Can you work these out from the model? Positions are in its coordinate system, mm. Face numbers are marked on the shaded views. A direction names the side the tool comes from. Give positions to 0.01 mm unless a question says otherwise; leave off trailing zeros. Order: outer loops, then holes, each group sorted by start corner. A loop starts at its lowest first (then second) coordinate and runs counter-clockwise, first axis right, second up. Notation, with made-up numbers: (-7.5, 55) - (43.5, 55) arc R34 ccw to (43.5, 87) - close; hole circle Ø9 at (44.25, 56). An arc over 180 degrees is marked (long way). Return JSON: item names as keys, results as strings.
Autodesk Inventor part; units mm, degrees
ref_plane "YZ Plane" through (0, 0, 0) normal (1, 0, 0) x (0, 1, 0)
ref_plane "XZ Plane" through (0, 0, 0) normal (0, 1, 0) x (-1, 0, 0)
ref_plane "XY Plane" through (0, 0, 0) normal (0, 0, 1) x (1, 0, 0)
sketch "Sketch1" plane through (0, 0, 0) normal (0, 0, 1) x (1, 0, 0)
  circle A0 centre (50.3282, 23.2015) radius 3
  circle A1 centre (18.8282, 23.2015) radius 3
  circle A2 centre (34.5782, 23.2015) radius 4
  arc A3 (37.4648, 32.7758) -> (30.5806, 32.3677) centre (34.5782, 23.2015) ccw
  arc A4 (50.3282, 17.7015) -> (51.8996, 28.4722) centre (50.3282, 23.2015) ccw
  line L0 (37.4648, 32.7758) -> (51.8996, 28.4722)
  line L1 (34.3282, 9.7015) -> (44.1532, 9.7015)
  line L2 (44.1532, 9.7015) -> (44.1532, 16.7015)
  line L3 (44.1532, 16.7015) -> (50.3282, 17.7015)
  line L4 (30.5806, 32.3677) -> (17.2831, 28.48)
  line L5 (34.3282, 9.7015) -> (25.0032, 9.7015)
  line L6 (25.0032, 9.7015) -> (25.0032, 16.7015)
  line L7 (25.0032, 16.7015) -> (18.8282, 17.7015)
  arc A5 (17.2831, 28.48) -> (18.8282, 17.7015) centre (18.8282, 23.2015) ccw
  circle A6 centre (34.5782, 23.2015) radius 8.7313
  point P0 (0, 0)
  dimension "d0" = 31.5
  dimension "d1" = 6
  dimension "d2" = 8
  dimension "d3" = 15.75
  dimension "d4" = 20
  dimension "d5" = 11
  dimension "d7" = 9.825
  dimension "d8" = 7
  dimension "d9" = 11
  dimension "d12" = 17.4625
  dimension "d14" = 0
extrude "Extrusion1" add sketch "Sketch1" along normal blind 10 contours L0 A4 L3 L2 L1 L5 L6 L7 A5 L4 A3 | A6
properties part number "shaft support"
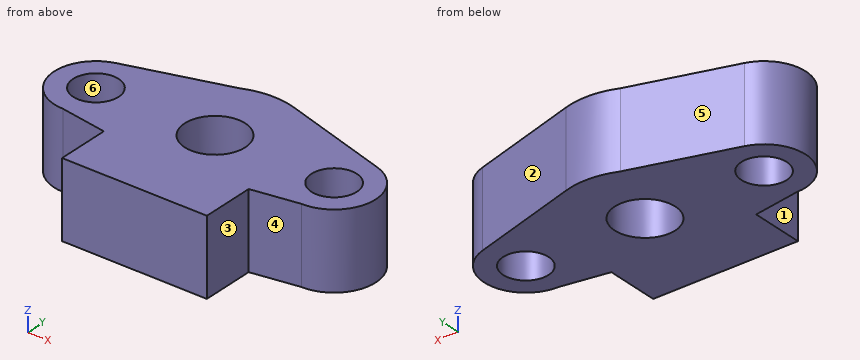
1. Thinking about a two-plate mould opening in X: for the marked faces 4, 5 and 6, which applies, +X half, -X half, draft (parallel to the pull), parting line (faces both ways), or undercut?
Checks:
{"face 4": "+X half", "face 5": "-X half", "face 6": "undercut"}
2. Suppose I cut it at D-D (y = 14.25). List the corners of the cut face in (x, z) for me.
Checks:
{"outline": "(25, 0) - (44.15, 0) - (44.15, 10) - (25, 10) - close"}
3. Suppose I cut it at C-C (y = 21.75). List the corners of the cut face in (x, z) for me, plus the area to 3 significant figures.
Checks:
{"outline": "(13.52, 0) - (16.2, 0) - (16.2, 10) - (13.52, 10) - close; (21.45, 0) - (30.85, 0) - (30.85, 10) - (21.45, 10) - close; (38.31, 0) - (47.7, 0) - (47.7, 10) - (38.31, 10) - close; (52.95, 0) - (55.63, 0) - (55.63, 10) - (52.95, 10) - close", "area": "242 mm^2"}
4. Suppose I cut it at B-B (z = 6). List the corners of the cut face in (x, y) for me, plus the area to 3 significant figures.
Checks:
{"outline": "(17.28, 28.48) arc R5.5 ccw to (18.83, 17.7) - (25, 16.7) - (25, 9.7) - (44.15, 9.7) - (44.15, 16.7) - (50.33, 17.7) arc R5.5 ccw to (51.9, 28.47) - (37.46, 32.78) arc R10 ccw to (30.58, 32.37) - close; hole circle Ø6 at (18.83, 23.2); hole circle Ø8 at (34.58, 23.2); hole circle Ø6 at (50.33, 23.2)", "area": "574 mm^2"}
5. For pin 1 Ø5 at (y, z) = (29.5, 4) entering from +X; pin 2 Ø5.5 at (y, z) = (13, 7) entering from +X; pin 3 Ø5.5 at (y, z) = (12, 4.5) entering from -X, each with a flat end and sliding along its axis, tell me the tip position at first contact or that it passes through.
Checks:
{"pin 1": "x = 54.31", "pin 2": "x = 44.15", "pin 3": "x = 25"}
6. If I drill on L1, parallel to X at y = 23.25, z = 1; L2, parallel to X at y = 25, z = 4.5; L3, parallel to Y at x = 35, z = 8, over which ranges is the centre line in solid material (lowest first)? Write a range as [from, to].
Checks:
{"L1": "[13.33, 15.83], [21.83, 30.58], [38.58, 47.33], [53.33, 55.83]", "L2": "[13.63, 16.43], [21.23, 31.01], [38.15, 47.93], [52.73, 55.53]", "L3": "[9.7, 19.22], [27.18, 33.19]"}
7. Suppose I cut it at A-A (y = 24.75). List the corners of the cut face in (x, z) for me.
Checks:
{"outline": "(13.55, 0) - (16.26, 0) - (16.26, 10) - (13.55, 10) - close; (21.4, 0) - (30.89, 0) - (30.89, 10) - (21.4, 10) - close; (38.27, 0) - (47.76, 0) - (47.76, 10) - (38.27, 10) - close; (52.9, 0) - (55.61, 0) - (55.61, 10) - (52.9, 10) - close"}
8. On a 3-axis mill with a long thin cutter (end or side, diameter ignored), from which of +Z, -Z, +X, -X, +Y, -Y can I reach the whole of each face in a straight line? I mean the marked faces 1, 2 and 3. Say none if no direction works.
Checks:
{"face 1": "+Z, -Z, -X, -Y", "face 2": "+Z, -Z, +X, +Y", "face 3": "+Z, -Z, +X, -Y"}
